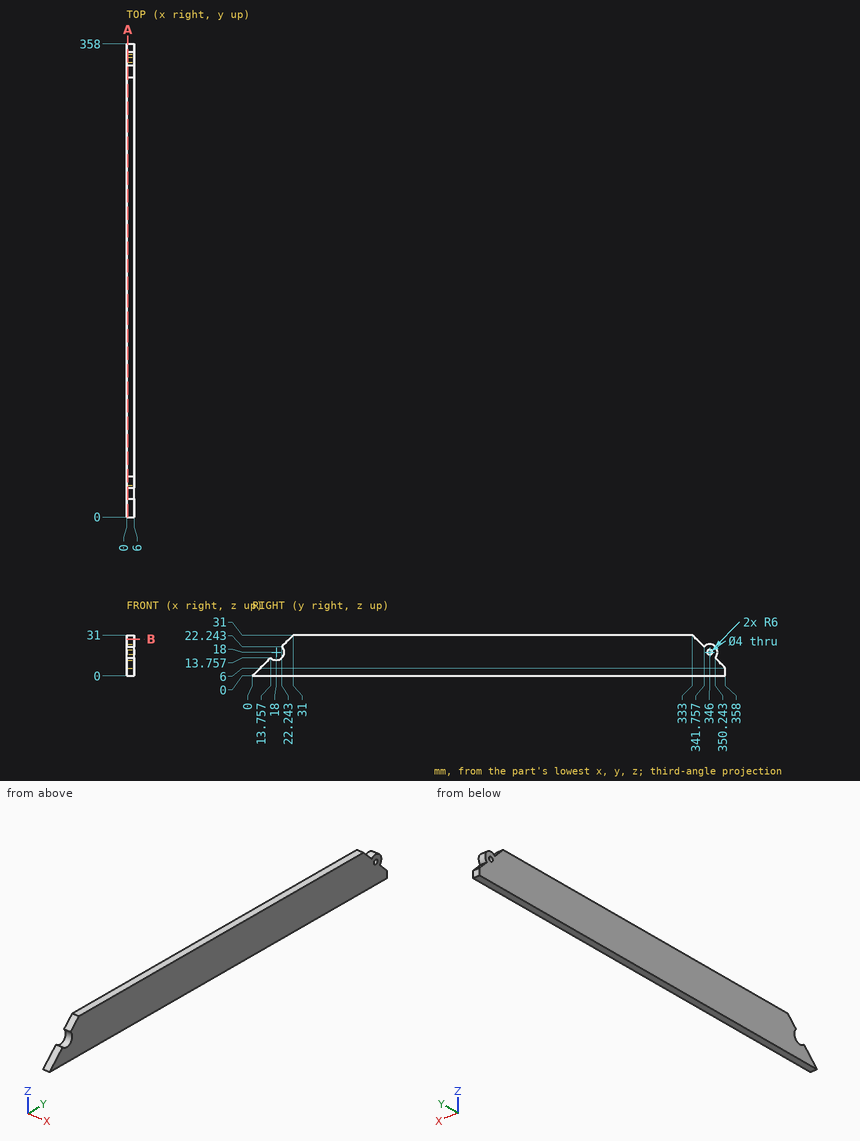
For this review, use the dimensioned drawing (mm, ordinates from the lowest corner) and the shaded views. Coordinates: 2 decimals unless noted, no trailing zeros. Order: outer loops, then holes, each group sorted by start corner. A loop starts at its lowest first (then second) coordinate and runs counter-clockwise, first axis right, second up. Notation, with made-up numbers: (-30.75, -2) -> (20.25, -2) arc R19 ccw to (20.25, 28) -> close; hole circle Ø3 at (84, 0). An arc over 180 degrees is marked (long way). One line per item, written item: value. Start each with the question number.
Q1. Take a section at B-B, the plane z = 28. State the section outline as (x, y) points.
Q2. Insertion check: pin 1 Ø3 at (x, z) = (5, 8.5) entering from -Y; pin 2 Ø1 at (x, z) = (4, 5.5) entering from -Y. Each pin has a flat end and moves straight along its axis. Give the tip position at first contact, or say it passes through.
Q3. Take a section at A-A, the plane x = 1.05. State the section outline as (y, z) points, then the cut area to 3 significant figures.
Q4. For probe 1 along Y at (x, z) = (2.5, 18); probe 2 along Z at (x, y) = (3.1, 346); probe 3 along Y at (x, z) = (4.15, 6), list the stretches that pass through material, from the lowest coordinate up.
Values follow:
1. outline: (0, 28) -> (6, 28) -> (6, 336) -> (0, 336) -> close
2. pin 1: stops at y = 7
2. pin 2: stops at y = 5
3. outline: (0, 0) -> (358, 0) -> (358, 6) -> (350.24, 13.76) arc R6 ccw to (341.76, 22.24) -> (333, 31) -> (31, 31) -> (22.24, 22.24) arc R6 cw to (13.76, 13.76) -> close; hole circle Ø4 at (346, 18)
3. area: 10,300 mm2
4. probe 1: y = 24 to 344, 348 to 352
4. probe 2: z = 0 to 16, 20 to 24
4. probe 3: y = 6 to 358
